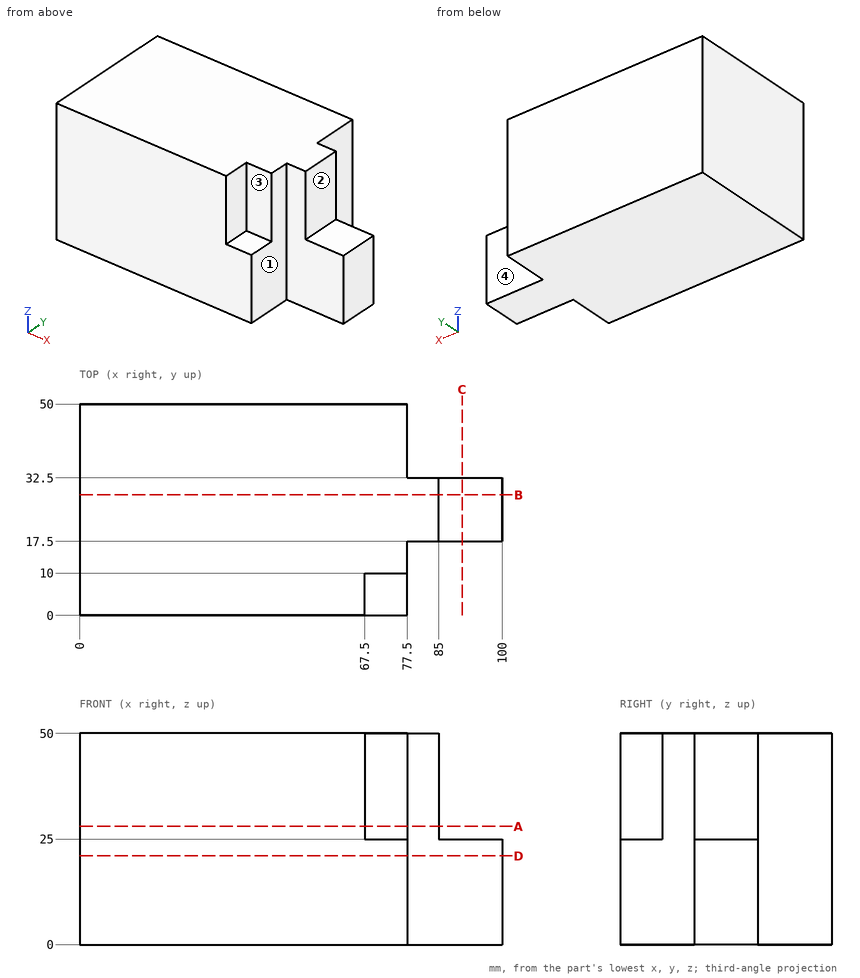
Source: three-view drawing plus pictorial views. Frame: mm from the lowest corner of the part. A direction names the side the tool comes from. Round coordinates to 2 decimals unless told otherwise and drop trailing zeros. Write each loop counter-clockwise with the first axis right and the second up, starting at its lowest first coordinate (ties: lowest second). Pieces come first, ordered by that corner, then holes. Notation, with made-up numbers: M 62.5,2.5 L 78.5,2.5 A35 cw 78.5,38.5 Z; hole C -37,76 d10. An arc over 180 degrees is marked long. Use CSV: the item, a comma, the result in double quotes. Start each with the question number.
Q1. Cut plane D-D on z = 21. Output: boundary loops of the cut face in (x, y), plus the area to 3 significant figures.
Q2. Line query: line 1 (X direction, y = 30, z = 40); line 2 (X direction, y = 6.5, z = 16); line 3 (Y direction, x = 82, z = 5.5). Output: solid intervals per line, ascending. Write a range as from..to.
Q3. Cut plane A-A on z = 28. Output: boundary loops of the cut face in (x, y).
Q4. First-contact query: P1, Ø16.5, axis at y = 25, z = 34, coming from the +X side; P2, Ø5, axis at y = 40, z = 32.5, coming from the +X side; P3, Ø6, axis at x = 86, z = 13, coming from the +Y side. Flat tips, straight axial feed; report the tip coordinate or a pass-through.
Q5. Access query for the marked faces 1, 2, 3 and 4. Directions: +Z, -Z, +X, -X, +Y, -Y. A direction counts if a zero-diameter tool reaches every point of the face in a straight line with its end or side. Return the directions, or none.
Q6. Cut plane C-C on x = 90.5. Output: boundary loops of the cut face in (y, z).
Q7. Cut plane B-B on y = 28.5. Output: boundary loops of the cut face in (x, z), plus the area to 4 significant figures.
Results found:
1,outline,"M 0,0 L 77.5,0 L 77.5,17.5 L 100,17.5 L 100,32.5 L 77.5,32.5 L 77.5,50 L 0,50 Z"
1,area,"4,210 mm^2"
2,line 1,"0..85"
2,line 2,"0..77.5"
2,line 3,"17.5..32.5"
3,outline,"M 0,0 L 67.5,0 L 67.5,10 L 77.5,10 L 77.5,17.5 L 85,17.5 L 85,32.5 L 77.5,32.5 L 77.5,50 L 0,50 Z"
4,P1,"x = 85"
4,P2,"x = 77.5"
4,P3,"y = 32.5"
5,face 1,"+Z, -Z, +X, -Y"
5,face 2,"+Z, +X, +Y, -Y"
5,face 3,"+Z, +X, -Y"
5,face 4,"+Z, -Z, +X, +Y"
6,outline,"M 17.5,0 L 32.5,0 L 32.5,25 L 17.5,25 Z"
7,outline,"M 0,0 L 100,0 L 100,25 L 85,25 L 85,50 L 0,50 Z"
7,area,"4,625 mm^2"
